The listing builds one solid part. Answer for the finished solid, in the listing's coordinates (mm). A direction names the side the tool comes from. Coordinates: 2 decimals unless noted, no trailing zeros. Loops run counter-clockwise (first coordinate to the right, second up) from the corner with the lowest first, then second, coordinate; pieces in that order, holes last. Notation, with made-up numbers: (30.5, -7) -> (50.5, -7) arc R24 cw to (50.5, 22) -> close; hole circle Ø2 at (81, 42.25). An arc over 180 degrees is marked (long way). Answer in a Markdown table with one row per item.
```python
from build123d import *

# Parameters (mm, degrees)
SKETCH3_R               = 2.8
CUT_EXTRUDE2_DEPTH      = 3.25
CUT_EXTRUDE3_DEPTH      = 2
CUT_EXTRUDE4_DEPTH      = 188.637949253
CUT_EXTRUDE4_DEPTH_BACK = 188.637949253
SKETCH5_R               = 8.25
CUT_EXTRUDE5_DEPTH      = 115.087685576
CUT_EXTRUDE5_DEPTH_BACK = 115.087685576
SKETCH6_W               = 80.378885923
SKETCH6_H               = 187.007266033


with BuildPart() as part:
    # Sketch1 → Revolve1 (revolve)
    with BuildSketch(Plane(origin=(0, 0, 0), x_dir=(0, 0, -1), z_dir=(1, 0, 0)), mode=Mode.PRIVATE) as revolve1_sk:
        Polygon((-76, 0), (124.5, 0), (124.5, 4), (109, 4), (109, 8), (108, 8), (108, 24), (104, 24), (104, 25), (0, 25), (0, 26), (-50, 26), (-50, 9), (-52, 9), (-52, 6), (-76, 6), align=None)
    revolve(revolve1_sk.sketch.rotate(Axis((0, 0, 76), (0, 0, -1)), 180), axis=Axis((0, 0, 76), (0, 0, -1)))

    # Sketch3 → Cut-Extrude2 (cut)
    with BuildSketch(Plane.XY.offset(-108)):
        with Locations(Location((6.767859423, 19.032500593, 0), (0, 0, 180))):
            Circle(SKETCH3_R)
        with Locations(Location((-19.905985431, 3.433910891, 0), (0, 0, 180))):
            Circle(SKETCH3_R)
        with Locations(Location((0, -20.2, 0), (0, 0, 180))):
            Circle(SKETCH3_R)
    extrude(amount=CUT_EXTRUDE2_DEPTH, mode=Mode.SUBTRACT)

    # Sketch4 → Cut-Extrude3 (cut)
    with BuildSketch(Plane(origin=(0, 0, -108), x_dir=(-1, 0, 0), z_dir=(0, 0, -1))):
        Polygon((-22.506441861, -8.334271099), (-16.973308635, -2.811902197), (-2.844949371, -16.967800773), (-8.378082597, -22.490169675), (-11.338488517, -25.444816332), (-25.466847781, -11.288917756), align=None)
    extrude(amount=-CUT_EXTRUDE3_DEPTH, mode=Mode.SUBTRACT)

    # Sketch5 → Cut-Extrude4 (cut, two sides: drawn at the far end of the back side and taken through both)
    with BuildSketch(Plane(origin=(0, 0, -108), x_dir=(-1, 0, 0), z_dir=(0, 0, -1)).offset(-CUT_EXTRUDE4_DEPTH_BACK)):
        with Locations(Location((0, 0, 0), (0, 0, 90))):
            Circle(SKETCH5_R)
    extrude(amount=CUT_EXTRUDE4_DEPTH + CUT_EXTRUDE4_DEPTH_BACK, mode=Mode.SUBTRACT)

    # Sketch6 → Cut-Extrude5 (cut, two sides: drawn at the far end of the back side and taken through both)
    with BuildSketch(Plane(origin=(0, 0, 0), x_dir=(1, 0, 0), z_dir=(0, 1, 0)).offset(-CUT_EXTRUDE5_DEPTH_BACK)):
        with Locations((-2.527125216, 13.496366983)):
            Rectangle(SKETCH6_W, SKETCH6_H)
    extrude(amount=CUT_EXTRUDE5_DEPTH + CUT_EXTRUDE5_DEPTH_BACK, mode=Mode.SUBTRACT)


solid = part.part
```
Item 1: A cutting plane is placed at C-C, the plane x = -6. Determine the outline of the cut face in (y, z).
Findings below:
| item | result |
|---|---|
| outline | (-23.24, -108) -> (-5.66, -108) -> (-5.66, -107) -> (-23.24, -107) -> close; (5.66, -108) -> (23.24, -108) -> (23.24, -107) -> (5.66, -107) -> close |
Item 2: A cutting plane is placed at D-D, the plane z = -107.35. Determine the outline of the cut face in (x, y).
Findings below:
| item | result |
|---|---|
| outline | (2.84, -16.97) -> (16.97, -2.81) -> (22.51, -8.33) arc R24 ccw (long way) to (8.38, -22.49) -> close; hole circle Ø5.6 at (-19.91, 3.43); hole circle Ø16.5 at (0, 0); hole circle Ø5.6 at (0, -20.2); hole circle Ø5.6 at (6.77, 19.03) |
Item 3: Find the intervals of material crossed by probe 1 along Y at (x, z) = (0, -107.8); probe 2 along X at (y, z) = (3.5, -107.05); probe 3 along Y at (x, z) = (3, -107.45), in increasing order.
Findings below:
| item | result |
|---|---|
| probe 1 | y = -24 to -23, -17.4 to -8.25, 8.25 to 24 |
| probe 2 | x = -23.74 to -22.71, -17.11 to -7.47, 7.47 to 23.74 |
| probe 3 | y = -23.81 to -17.12, -16.81 to -7.69, 7.69 to 23.81 |
Item 4: A cutting plane is placed at A-A, the plane x = 0. Determine the outline of the cut face in (y, z), plus the area to 3 significant figures.
Findings below:
| item | result |
|---|---|
| outline | (-24, -108) -> (-23, -108) -> (-23, -107) -> (-24, -107) -> close; (-17.4, -108) -> (-8.25, -108) -> (-8.25, -107) -> (-17.4, -107) -> close; (8.25, -108) -> (24, -108) -> (24, -107) -> (8.25, -107) -> close |
| area | 25.9 mm2 |
Item 5: Determine the mould class of faces 3 (the face through (5.57, -19.69, -107.51)), 4 (the face through (19.779, -5.612, -107.507)), 5 (the face through (-8.054, -1.788, -107.493)), 6 (the face through (0, 10, -108)) for opening direction X: +X half, -X half, draft (parallel to the pull), parting line (faces both ways), or undercut.
Findings below:
| item | result |
|---|---|
| face 3 | +X half |
| face 4 | undercut |
| face 5 | undercut |
| face 6 | draft |
Item 6: A flat-ended cylindrical pin translates along its axis: pin 1 Ø5 at (x, y) = (-19.91, 3.43) entering from +Z. Find the tip coordinate at first contact, or state that the pin passes through.
Findings below:
| item | result |
|---|---|
| pin 1 | passes through |
Item 7: A tool of negligible diameter and unlimited length cuts with its end or side. For faces 1 (the face through (0, 10, -107)), 2 (the face through (10, -9.8, -107.5)), from which of +Z, -Z, +X, -X, +Y, -Y can it reach the whole face along a straight path? Write none if from no direction.
Findings below:
| item | result |
|---|---|
| face 1 | +Z, +X, -X, +Y, -Y |
| face 2 | +Z, -Z |
Item 8: A cutting plane is placed at B-B, the plane y = 0. Determine the outline of the cut face in (x, z), plus the area to 3 significant figures.
Findings below:
| item | result |
|---|---|
| outline | (-24, -108) -> (-8.25, -108) -> (-8.25, -107) -> (-24, -107) -> close; (8.25, -108) -> (24, -108) -> (24, -107) -> (8.25, -107) -> close |
| area | 31.5 mm2 |
